```python
from build123d import *

# Parameters (mm, degrees)
SKETCH1_R           = 15
BOSS_EXTRUDE1_DEPTH = 5
SKETCH2_R           = 2
BOSS_EXTRUDE2_DEPTH = 15
FILLET1_R           = 6
SKETCH3_R           = 1.5
CUT_EXTRUDE1_DEPTH  = 26.980762114
CIRPATTERN1_COUNT   = 3


with BuildPart() as part:
    # Sketch1 → Boss-Extrude1 (new body)
    with BuildSketch(Plane(origin=(0, 0, 0), x_dir=(1, 0, 0), z_dir=(0, 1, 0))):
        with Locations(Location((0, 0, 0), (0, 0, 270))):
            Circle(SKETCH1_R)
    extrude(amount=BOSS_EXTRUDE1_DEPTH)

    # Sketch2 → Boss-Extrude2 (add)
    with BuildSketch(Plane(origin=(0, 5, 0), x_dir=(1, 0, 0), z_dir=(0, 1, 0))):
        with Locations(Location((0, 0, 0), (0, 0, 270))):
            Circle(SKETCH2_R)
    extrude(amount=BOSS_EXTRUDE2_DEPTH)

    # Fillet1
    fillet1_edges = [part.edges().sort_by_distance(p)[0] for p in [
        (0, 5, -2),
    ]]
    fillet(fillet1_edges, radius=FILLET1_R)

    # Sketch3 → Cut-Extrude1 (cut, through all)
    with BuildSketch(Plane(origin=(0, 5, 0), x_dir=(1, 0, 0), z_dir=(0, 1, 0))):
        with Locations(Location((-2.532093929, -11.72981246, 0), (0, 0, 270))):
            Circle(SKETCH3_R)
    cut_extrude1 = extrude(amount=-CUT_EXTRUDE1_DEPTH, mode=Mode.SUBTRACT)

    # CirPattern1: Cut-Extrude1 ×3 about axis
    cirpattern1_axis = Axis((0, 0, 0), (0, 1, 0))
    for i in range(1, CIRPATTERN1_COUNT):
        add(cut_extrude1.rotate(cirpattern1_axis, i * 360 / CIRPATTERN1_COUNT), mode=Mode.SUBTRACT)


solid = part.part
```
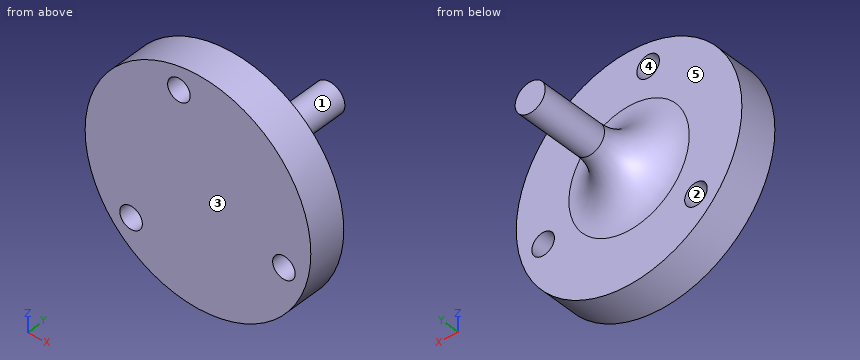
Can you work these out from the model? Positions are in its coordinate system, mm. Face numbers are marked on the shaded views. A direction names the side the tool comes from. Round coordinates to 2 decimals unless told otherwise and drop trailing zeros. Loops run counter-clockwise (first coordinate to the right, second up) from the corner with the lowest first, then second, coordinate; pieces in that order, holes last. Notation, with made-up numbers: M -10,6 L 45,6 A16 ccw 45,20 Z; hole C 44.5,20 d6. An arc over 180 degrees is marked long. Write item = value, one per line. Start each with the question number.
(1) Suppose I cut it at A-A on z = 0. Write out the boundary of the cut face in (x, y).
(2) Suppose I cut it at C-C on z = 12.75. Write out the boundary of the cut face in (x, y), plus the area to 3 significant figures.
(3) If we mould it in two halves opening along Z, with no side actions, what happens to the marked faces 1, 2 and 3? For each: released by +Z, released by -Z, zero draft, split by the parting line, or undercut.
(4) I'm going to push flat-ended pins straight in: P1, Ø2, axis at y = 7, z = -1.5, coming from the -X side; P2, Ø4, axis at x = 11.42, z = -3.67, coming from the +Y side; P3, Ø1.5, axis at x = -2, y = 15.5, coming from the +Z side. Where does each tip first touch, or does it pass through?
(5) I need wall thicknesses on line 1 along X through (y, z) = (3, 10.75); line 2 along Z through (x, y) = (-3.75, 4.75); line 3 along X through (y, z) = (2.5, -2.5). Which ranges of each line are inside material? Lowest first, please.
(6) Which directions (+Z, -Z, +X, -X, +Y, -Y) give clear straight access to the entire face, cutting with the end or side of a thin tool? Please do the marked faces 4 and 5.
(7) Suppose I cut it at D-D on x = 0. Write out the boundary of the cut face in (y, z).
(8) Suppose I cut it at B-B on x = 11.5. Write out the boundary of the cut face in (y, z).
Answer block:
q1.outline = M -15,0 L 15,0 L 15,5 L 8,5 A6 cw 2,11 L 2,20 L -2,20 L -2,11 A6 cw -8,5 L -15,5 Z
q2.outline = M -7.9,0 L -3.63,0 L -3.63,5 L -7.9,5 Z; M -1.43,0 L 7.9,0 L 7.9,5 L -1.43,5 Z
q2.area = 68.0 mm²
q3.face_1 = split by the parting line
q3.face_2 = undercut
q3.face_3 = zero draft
q4.P1 = -4.47
q4.P2 = 5
q4.P3 = 1.56
q5.line_1 = -10.46 to -3.67, -1.4 to 10.46
q5.line_2 = -14.52 to 10.85, 12.61 to 14.52
q5.line_3 = -14.79 to 10.49, 12.36 to 14.79
q6.face_4 = +Y, -Y
q6.face_5 = +Y
q7.outline = M 0,-15 L 5,-15 L 5,-8 A6 cw 11,-2 L 20,-2 L 20,2 L 11,2 A6 cw 5,8 L 5,15 L 0,15 Z
q8.outline = M 0,-9.63 L 5,-9.63 L 5,-5.17 L 0,-5.17 Z; M 0,-2.17 L 5,-2.17 L 5,9.63 L 0,9.63 Z
